Model file for the job. Use its own axes, mm. A direction names the side the tool comes from. Coordinates: 2 decimals unless noted, no trailing zeros. Write each loop counter-clockwise with the first axis right and the second up, starting at its lowest first coordinate (ties: lowest second). Pieces come first, ordered by that corner, then holes. Notation, with made-up numbers: M 13.5,59 L 62.5,59 A23 ccw 62.5,97 Z; hole C 41,-26 d2. An arc over 180 degrees is marked long. Answer in a Markdown table with one row per item. Add a question column.
```python
from build123d import *

# Parameters (mm, degrees)
F0_W     = 50.8
F0_H     = 25
F1_DEPTH = 1
F2_R     = 1.5
F3_DEPTH = 25
F5_DEPTH = 25


with BuildPart() as f1:
    # F0 (on Top) → F1 (new body)
    with BuildSketch(Plane.XY):
        Rectangle(F0_W, F0_H)
    extrude(amount=F1_DEPTH)

    # F2 (on face) → F3 (cut)
    with BuildSketch(Plane.XY.offset(1)):
        with Locations((19.516597, 3.062223)):
            Circle(F2_R)
    extrude(amount=-F3_DEPTH, mode=Mode.SUBTRACT)

    # F4 (on face) → F5 (cut)
    with BuildSketch(Plane.XY.offset(1)):
        Polygon((-4.253665, -6.413301), (-7.367644, -12.5), (-4.253665, -12.5), align=None)
        Polygon((2.443298, -6.413301), (-1.253027, -12.5), (2.443298, -12.5), align=None)
        Polygon((-9.930169, -6.413301), (-13.044149, -12.5), (-9.930169, -12.5), align=None)
    extrude(amount=-F5_DEPTH, mode=Mode.SUBTRACT)


solid = f1.part
```
1) Slice it at C-C (z = 0.2). Give the cut face in (x, y).
2) Slice it at B-B (x = 20.5). Give the cut face in (y, z), then the cut area to 3 significant figures.
3) Slice it at A-A (y = -8). Give the cut face in (x, z), then the cut area to 3 significant figures.
4) Two-plate mould, pull along Y, no slides. Class faces 1 (the face through (-0.4, 12.5, 0.5)), 2 (the face through (0, 0, 0)), 3 (the face through (-2.8, -12.5, 0.5)), 4 (the face through (19.32, 4.55, 0.51)): released by +Y, released by -Y, zero draft, split by the parting line, or undercut.
5) Which spindle directions (+Z, -Z, +X, -X, +Y, -Y) get a long thin tool onto all of the face, cutting with end or side? Do faces 5 (the face through (-25.4, -0.2, 0.5)), 6 (the face through (-5.789, -9.414, 0.507)). Say none if no direction does.
6) Drill centre lines: probe 1 along X at (y, z) = (-8.25, 0.4); probe 2 along X at (y, z) = (-8.75, 0.2); probe 3 along Y at (x, z) = (20.5, 0.9). Where is each one in solid material? Low to high.
7) Slice it at D-D (x = -12.5). Give the cut face in (y, z), then the cut area to 3 significant figures.
Ans:
| question | item | result |
|---|---|---|
| 1 | outline | M -25.4,-12.5 L -13.04,-12.5 L -9.93,-6.41 L -9.93,-12.5 L -7.37,-12.5 L -4.25,-6.41 L -4.25,-12.5 L -1.25,-12.5 L 2.44,-6.41 L 2.44,-12.5 L 25.4,-12.5 L 25.4,12.5 L -25.4,12.5 Z; hole C 19.52,3.06 d3 |
| 2 | outline | M -12.5,0 L 1.93,0 L 1.93,1 L -12.5,1 Z; M 4.19,0 L 12.5,0 L 12.5,1 L 4.19,1 Z |
| 2 | area | 22.7 mm2 |
| 3 | outline | M -25.4,0 L -10.74,0 L -10.74,1 L -25.4,1 Z; M -9.93,0 L -5.07,0 L -5.07,1 L -9.93,1 Z; M -4.25,0 L 1.48,0 L 1.48,1 L -4.25,1 Z; M 2.44,0 L 25.4,0 L 25.4,1 L 2.44,1 Z |
| 3 | area | 48.2 mm2 |
| 4 | face 1 | released by +Y |
| 4 | face 2 | zero draft |
| 4 | face 3 | released by -Y |
| 4 | face 4 | undercut |
| 5 | face 5 | +Z, -Z, -X, +Y, -Y |
| 5 | face 6 | +Z, -Z, -Y |
| 6 | probe 1 | x = -25.4 to -10.87, -9.93 to -5.19, -4.25 to 1.33, 2.44 to 25.4 |
| 6 | probe 2 | x = -25.4 to -11.13, -9.93 to -5.45, -4.25 to 1.02, 2.44 to 25.4 |
| 6 | probe 3 | y = -12.5 to 1.93, 4.19 to 12.5 |
| 7 | outline | M -11.44,0 L 12.5,0 L 12.5,1 L -11.44,1 Z |
| 7 | area | 23.9 mm2 |
